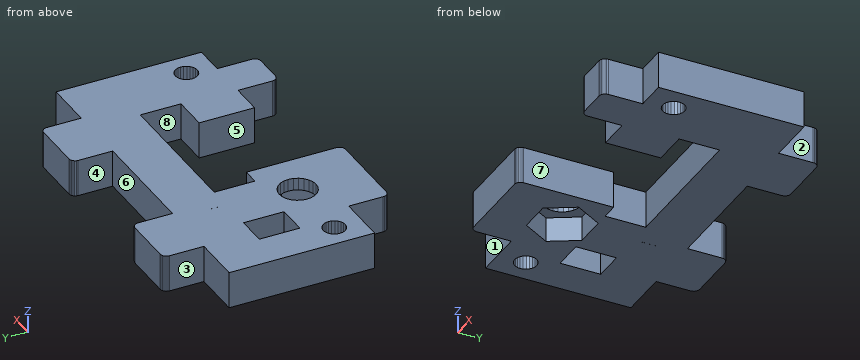
from build123d import *

# Parameters (mm, degrees)
BOSS_EXTRUDE1_DEPTH = 6
BOSS_EXTRUDE2_DEPTH = 2


with BuildPart() as part:
    # Sketch1 → Boss-Extrude1 (new body)
    with BuildSketch(Plane.XY):
        Polygon((-427.525990336, -199.228814306), (-427.367071713, -199.021707525), (-427.267171291, -198.78052657), (-427.233097117, -198.521707525), (-427.233097117, -183.921707525), (-429.945372541, -183.921707525), (-429.945372541, -177.321707525), (-406.445372541, -177.321707525), (-406.445372541, -183.921707525), (-412.227908952, -183.921707525), (-412.227908952, -192.921707525), (-406.945372541, -192.921707525), (-406.945372541, -198.521707525), (-406.911298367, -198.78052657), (-406.811397945, -199.021707525), (-406.652479322, -199.228814306), (-406.445372541, -199.387732928), (-406.204191586, -199.487633351), (-405.945372541, -199.521707525), (-401.345372541, -199.521707525), (-401.086553496, -199.487633351), (-400.845372541, -199.387732928), (-400.63826576, -199.228814306), (-400.479347137, -199.021707525), (-400.379446715, -198.78052657), (-400.345372541, -198.521707525), (-400.345372541, -192.921707525), (-395.345372541, -192.921707525), (-395.345372541, -169.321707525), (-403.345372541, -169.321707525), (-403.345372541, -163.721707525), (-403.379446715, -163.46288848), (-403.479347137, -163.221707525), (-403.63826576, -163.014600744), (-403.845372541, -162.855682121), (-404.086553496, -162.755781698), (-404.345372541, -162.721707525), (-412.345372541, -162.721707525), (-412.604191586, -162.755781698), (-412.845372541, -162.855682121), (-413.052479322, -163.014600744), (-413.211397945, -163.221707525), (-413.311298367, -163.46288848), (-413.345372541, -163.721707525), (-413.345372541, -169.321707525), (-432.345372541, -169.321707525), (-432.345372541, -163.721707525), (-432.379446715, -163.46288848), (-432.479347137, -163.221707525), (-432.63826576, -163.014600744), (-432.845372541, -162.855682121), (-433.086553496, -162.755781698), (-433.345372541, -162.721707525), (-441.345372541, -162.721707525), (-441.604191586, -162.755781698), (-441.845372541, -162.855682121), (-442.052479322, -163.014600744), (-442.211397945, -163.221707525), (-442.311298367, -163.46288848), (-442.345372541, -163.721707525), (-442.345372541, -169.321707525), (-450.345372541, -169.321707525), (-450.345372541, -192.921707525), (-442.145372541, -192.921707525), (-442.145372541, -198.521707525), (-442.111298367, -198.78052657), (-442.011397945, -199.021707525), (-441.852479322, -199.228814306), (-441.645372541, -199.387732928), (-441.404191586, -199.487633351), (-441.145372541, -199.521707525), (-428.233097117, -199.521707525), (-427.974278072, -199.487633351), (-427.733097117, -199.387732928), align=None)
        Polygon((-439.240180663, -183.921707525), (-439.245372541, -177.321707525), (-444.245370992, -177.325642806), (-444.240179116, -183.925640764), align=None, mode=Mode.SUBTRACT)
        Polygon((-447.245372541, -186.862861798), (-447.618164747, -187.148915319), (-447.904218268, -187.521707525), (-448.084039028, -187.955833244), (-448.145372541, -188.421707525), (-448.084039028, -188.887581806), (-447.904218268, -189.321707525), (-447.618164747, -189.694499731), (-447.245372541, -189.980553252), (-446.811246822, -190.160374012), (-446.345372541, -190.221707525), (-445.87949826, -190.160374012), (-445.445372541, -189.980553252), (-445.072580335, -189.694499731), (-444.786526814, -189.321707525), (-444.606706054, -188.887581806), (-444.545372541, -188.421707525), (-444.606706054, -187.955833244), (-444.786526814, -187.521707525), (-445.072580335, -187.148915319), (-445.445372541, -186.862861798), (-445.87949826, -186.683041037), (-446.345372541, -186.621707525), (-446.811246822, -186.683041037), align=None, mode=Mode.SUBTRACT)
        Polygon((-400.618164747, -187.148915319), (-400.904218268, -187.521707525), (-401.084039028, -187.955833244), (-401.145372541, -188.421707525), (-401.084039028, -188.887581806), (-400.904218268, -189.321707525), (-400.618164747, -189.694499731), (-400.245372541, -189.980553252), (-399.811246822, -190.160374012), (-399.345372541, -190.221707525), (-398.87949826, -190.160374012), (-398.445372541, -189.980553252), (-398.072580335, -189.694499731), (-397.786526814, -189.321707525), (-397.606706054, -188.887581806), (-397.545372541, -188.421707525), (-397.606706054, -187.955833244), (-397.786526814, -187.521707525), (-398.072580335, -187.148915319), (-398.445372541, -186.862861798), (-398.87949826, -186.683041037), (-399.345372541, -186.621707525), (-399.811246822, -186.683041037), (-400.245372541, -186.862861798), align=None, mode=Mode.SUBTRACT)
        Polygon((-437.308125833, -192.934124647), (-432.11197341, -192.934124647), (-429.513897199, -188.434124647), (-432.11197341, -183.934124647), (-437.308125833, -183.934124647), (-439.906202044, -188.434124647), align=None, mode=Mode.SUBTRACT)
        Polygon((-433.771349426, -176.175776495), (-433.791446368, -176.271985766), (-433.771349426, -172.366944559), align=None, mode=Mode.SUBTRACT)
    extrude(amount=-BOSS_EXTRUDE1_DEPTH)

    # Sketch1_3 → Boss-Extrude2 (add)
    with BuildSketch(Plane.XY):
        Polygon((-437.308125833, -192.934124647), (-432.11197341, -192.934124647), (-429.513897199, -188.434124647), (-432.11197341, -183.934124647), (-437.308125833, -183.934124647), (-439.906202044, -188.434124647), align=None)
        Polygon((-437.192655779, -192.734124647), (-432.227443464, -192.734124647), (-429.744837306, -188.434124647), (-432.227443464, -184.134124647), (-437.192655779, -184.134124647), (-439.675261936, -188.434124647), align=None, mode=Mode.SUBTRACT)
        Polygon((-439.675261936, -188.434124647), (-437.192655779, -192.734124647), (-432.227443464, -192.734124647), (-429.744837306, -188.434124647), (-432.227443464, -184.134124647), (-437.192655779, -184.134124647), align=None)
        Polygon((-439.444321829, -188.434124647), (-437.077185725, -192.534124647), (-432.342913518, -192.534124647), (-429.975777414, -188.434124647), (-432.342913518, -184.334124647), (-437.077185725, -184.334124647), align=None, mode=Mode.SUBTRACT)
        Polygon((-437.077185725, -184.334124647), (-439.444321829, -188.434124647), (-437.077185725, -192.534124647), (-432.342913518, -192.534124647), (-429.975777414, -188.434124647), (-432.342913518, -184.334124647), align=None)
        Polygon((-439.213381721, -188.434124647), (-436.961715671, -192.334124647), (-432.458383571, -192.334124647), (-430.206717522, -188.434124647), (-432.458383571, -184.534124647), (-436.961715671, -184.534124647), align=None, mode=Mode.SUBTRACT)
        Polygon((-436.961715671, -184.534124647), (-439.213381721, -188.434124647), (-436.961715671, -192.334124647), (-432.458383571, -192.334124647), (-430.206717522, -188.434124647), (-432.458383571, -184.534124647), align=None)
        Polygon((-432.573853625, -184.734124647), (-436.846245617, -184.734124647), (-438.982441613, -188.434124647), (-436.846245617, -192.134124647), (-432.573853625, -192.134124647), (-430.437657629, -188.434124647), align=None, mode=Mode.SUBTRACT)
        Polygon((-430.437657629, -188.434124647), (-432.573853625, -184.734124647), (-436.846245617, -184.734124647), (-438.982441613, -188.434124647), (-436.846245617, -192.134124647), (-432.573853625, -192.134124647), align=None)
        Polygon((-432.689323679, -191.934124647), (-430.668597737, -188.434124647), (-432.689323679, -184.934124647), (-436.730775563, -184.934124647), (-438.751501506, -188.434124647), (-436.730775563, -191.934124647), align=None, mode=Mode.SUBTRACT)
        Polygon((-436.730775563, -191.934124647), (-432.689323679, -191.934124647), (-430.668597737, -188.434124647), (-432.689323679, -184.934124647), (-436.730775563, -184.934124647), (-438.751501506, -188.434124647), align=None)
        Polygon((-432.804793733, -191.734124647), (-430.899537845, -188.434124647), (-432.804793733, -185.134124647), (-436.61530551, -185.134124647), (-438.520561398, -188.434124647), (-436.61530551, -191.734124647), align=None, mode=Mode.SUBTRACT)
        Polygon((-436.61530551, -191.734124647), (-432.804793733, -191.734124647), (-430.899537845, -188.434124647), (-432.804793733, -185.134124647), (-436.61530551, -185.134124647), (-438.520561398, -188.434124647), align=None)
        Polygon((-432.920263787, -191.534124647), (-431.130477952, -188.434124647), (-432.920263787, -185.334124647), (-436.499835456, -185.334124647), (-438.28962129, -188.434124647), (-436.499835456, -191.534124647), align=None, mode=Mode.SUBTRACT)
        Polygon((-436.499835456, -191.534124647), (-432.920263787, -191.534124647), (-431.130477952, -188.434124647), (-432.920263787, -185.334124647), (-436.499835456, -185.334124647), (-438.28962129, -188.434124647), align=None)
        Polygon((-437.727908952, -188.421707525), (-437.625686431, -189.19816466), (-437.325985163, -189.921707525), (-436.849229296, -190.543027868), (-436.227908952, -191.019783736), (-435.504366087, -191.319485004), (-434.727908952, -191.421707525), (-433.951451817, -191.319485004), (-433.227908952, -191.019783736), (-432.606588608, -190.543027868), (-432.129832741, -189.921707525), (-431.830131473, -189.19816466), (-431.727908952, -188.421707525), (-431.830131473, -187.645250389), (-432.129832741, -186.921707525), (-432.606588608, -186.300387181), (-433.227908952, -185.823631313), (-433.951451817, -185.523930046), (-434.727908952, -185.421707525), (-435.504366087, -185.523930046), (-436.227908952, -185.823631313), (-436.849229296, -186.300387181), (-437.325985163, -186.921707525), (-437.625686431, -187.645250389), align=None, mode=Mode.SUBTRACT)
    extrude(amount=-BOSS_EXTRUDE2_DEPTH)


solid = part.part
Here's how the part is built. I have some questions about the finished solid (model axes, mm). Face numbers are marked on the shaded views. A direction names the side the tool comes from. Coordinates: 2 decimals unless noted, no trailing zeros. Loops run counter-clockwise (first coordinate to the right, second up) from the corner with the lowest first, then second, coordinate; pieces in that order, holes last.
1. If we mould it in two halves opening along Y, with no side actions, what happens to the marked faces 6, 7 and 8? For each: pulls with the +Y half, pulls with the -Y half, needs draft (parallel to the pull), parting line crosses it, or undercut.
2. Imagine slicing it at B-B, the plane x = -426. Please give me the cut outline in (y, z), and give its area (3 significant figures).
3. For the marked faces 1, 2, 3, 4 and 5, which set-ups out of +Z, -Z, +X, -X, +Y, -Y let a thin tool reach every point of the face, with its end or its side?
4. For P1, Ø1.5, axis at x = -422, z = -2, coming from the -Y side; P2, Ø1.8, axis at x = -446.5, z = -4, coming from the -Y side; P3, Ø3, axis at y = -196.5, z = -4, coming from the -X side, each with a flat end and sliding along its axis, tell me the tip position at first contact or that it passes through.
5. Imagine slicing it at C-C, the plane y = -182.5. Please give me the cut outline in (x, z).
6. Imagine slicing it at D-D, the plane z = -3.25. Count the separate pieces of the cut face and the enclosed holes in it, and give its area (3 significant figures).
7. I need wall thicknesses on L1, parallel to X at y = -182, z = -4.2; L2, parallel to X at y = -192.5, z = -5.5; L3, parallel to X at y = -188, z = -2.05. Which ranges of each line are inside material? Lowest first, please.
8. Imagine slicing it at A-A, the plane y = -194. Please give me the cut outline in (x, z), and give its area (3 significant figures).
Taken from the geometry:
1. face 6: pulls with the +Y half
1. face 7: needs draft
1. face 8: undercut
2. outline: (-177.32, -6) - (-169.32, -6) - (-169.32, 0) - (-177.32, 0) - close
2. area: 48.0 mm2
3. face 1: +Z, -Z, -X, -Y
3. face 2: +Z, -Z, +X, +Y
3. face 3: +Z, -Z, -X, +Y
3. face 4: +Z, -Z, +Y
3. face 5: +Z, -Z, -Y
4. P1: stops at y = -177.32
4. P2: stops at y = -192.92
4. P3: stops at x = -442.15
5. outline: (-450.35, -6) - (-444.24, -6) - (-444.24, 0) - (-450.35, 0) - close; (-439.24, -6) - (-429.95, -6) - (-429.95, 0) - (-439.24, 0) - close; (-406.45, -6) - (-395.35, -6) - (-395.35, 0) - (-406.45, 0) - close
6. separate pieces: 1
6. enclosed holes: 5
6. area: 1,160 mm2
7. L1: x = -450.35 to -444.24, -439.24 to -429.95, -406.45 to -395.35
7. L2: x = -450.35 to -437.56, -431.86 to -427.23, -412.23 to -395.35
7. L3: x = -450.35 to -448.09, -444.6 to -439.66, -429.76 to -427.23, -412.23 to -401.09, -397.6 to -395.35
8. outline: (-442.15, -6) - (-427.23, -6) - (-427.23, 0) - (-442.15, 0) - close; (-406.95, -6) - (-400.35, -6) - (-400.35, 0) - (-406.95, 0) - close
8. area: 129 mm2
